Part model, mm, in its own coordinate system. Face numbers are marked on the shaded views. A direction names the side the tool comes from. Give positions to 0.01 mm unless a question says otherwise; leave off trailing zeros. Write each loop counter-clockwise with the first axis right and the second up, starting at its lowest first coordinate (ties: lowest second). Pieces come first, ordered by that corner, then holes.
```python
from build123d import *

# Parameters (mm, degrees)
PAD002_DEPTH    = 7
PAD003_DEPTH    = 3
CHAMFER003_SIZE = 1.5
SKETCH009_W     = 7.9
SKETCH009_H     = 8.3
PAD004_DEPTH    = 7.9
FILLET001_R     = 3.94
SKETCH010_R     = 1
HOLE002_DEPTH   = 25
SKETCH012_W     = 2.9
SKETCH012_H     = 8.3
PAD005_DEPTH    = 10
PAD006_DEPTH    = 8.3
FILLET002_R     = 0.5


with BuildPart() as part:
    # Sketch006 → Pad002 (new body)
    with BuildSketch(Plane.XY.offset(4)):
        Polygon((-62, 2.5), (-62, -16), (62, -16), (62, 2.5), (42, 2.5), (31.5, -8), (-31.5, -8), (-42, 2.5), align=None)
    extrude(amount=PAD002_DEPTH)

    # Sketch007 (on Face9 of Pad002) → Pad003 (join)
    with BuildSketch(Plane(origin=(0, 0, 4), x_dir=(1, 0, 0), z_dir=(0, 0, -1))):
        with BuildLine():
            Line((-31.5, 8), (31.5, 8))
            Line((37.293259, 2.206741), (31.5, 8))
            Line((38.566051, 3.479533), (37.293259, 2.206741))
            Line((32.772792, 9.272792), (38.566051, 3.479533))
            ThreePointArc((32.772792, 9.272792), (32.18883, 9.662983), (31.5, 9.8))
            Line((31.5, 9.8), (-31.5, 9.8))
            ThreePointArc((-31.5, 9.8), (-32.18883, 9.662983), (-32.772792, 9.272792))
            Line((-38.566051, 3.479533), (-32.772792, 9.272792))
            Line((-37.293259, 2.206741), (-38.566051, 3.479533))
            Line((-31.5, 8), (-37.293259, 2.206741))
        make_face()
    extrude(amount=PAD003_DEPTH)

    # Chamfer003
    chamfer003_edges = [part.edges().sort_by_distance(p)[0] for p in [
        (-35.669422, -6.376163, 4),
    ]]
    chamfer(chamfer003_edges, length=CHAMFER003_SIZE)

    # Sketch009 (on Face1 of Chamfer003) → Pad004 (join)
    with BuildSketch(Plane(origin=(0, 0, 4), x_dir=(1, 0, 0), z_dir=(0, 0, -1))):
        with Locations((-58.05, 6.75)):
            Rectangle(SKETCH009_W, SKETCH009_H)
    extrude(amount=PAD004_DEPTH)

    # Fillet001
    fillet001_edges = [part.edges().sort_by_distance(p)[0] for p in [
        (-54.1, -6.75, -3.9),
        (-62, -6.75, -3.9),
    ]]
    fillet(fillet001_edges, radius=FILLET001_R)

    # Sketch010 (on Face1 of Fillet001) → Hole002 (cut)
    with BuildSketch(Plane.XZ.offset(10.9)):
        with Locations((-58, 0)):
            Circle(SKETCH010_R)
    extrude(amount=-HOLE002_DEPTH, mode=Mode.SUBTRACT)

    # Sketch012 (on Face4 of Hole002) → Pad005 (join)
    with BuildSketch(Plane(origin=(0, 0, 4), x_dir=(1, 0, 0), z_dir=(0, 0, -1))):
        with Locations((60.55, 6.75)):
            Rectangle(SKETCH012_W, SKETCH012_H)
    extrude(amount=PAD005_DEPTH)

    # Sketch013 (on Face21 of Pad005) → Pad006 (join)
    with BuildSketch(Plane.XZ.offset(10.9)):
        Polygon((59.1, -6), (57.2, -2.1), (59.1, -2.1), align=None)
    extrude(amount=-PAD006_DEPTH)

    # Fillet002
    fillet002_edges = [part.edges().sort_by_distance(p)[0] for p in [
        (57.2, -6.75, -2.1),
    ]]
    fillet(fillet002_edges, radius=FILLET002_R)


solid = part.part
```
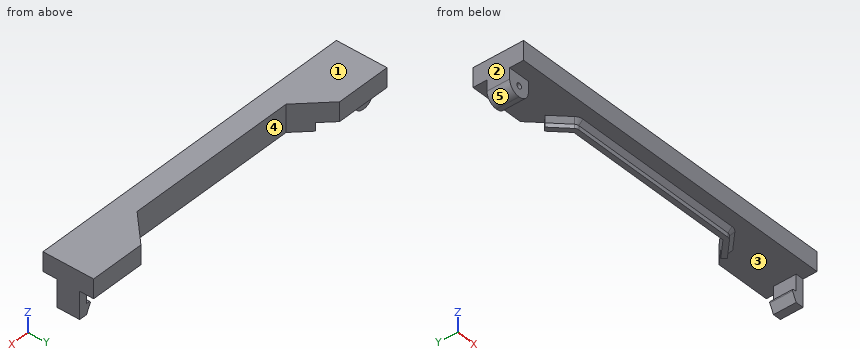
1) Pin check, flat tips, straight feed: pin 1 Ø3 at (y, z) = (-3, -3.5) entering from -X; pin 2 Ø4 at (x, z) = (-59.5, 1.5) entering from +Y; pin 3 Ø6 at (x, z) = (-35.5, 1) entering from +Y. Stop position of each tip, or through.
Answers follow:
pin 1: stops at x = -61.43
pin 2: stops at y = -2.6
pin 3: stops at y = -2.21
2) Wall check: L1, parallel to Z at x = -58, y = -4.25; L2, parallel to Y at x = -23.5, z = 9; L3, parallel to X at y = -7, z = 4.25. Give the ranges that are in metal, low to high.
Answers follow:
L1: z = -3.9 to -1, 1 to 11
L2: y = -16 to -8
L3: x = -62 to -32.5, 32.5 to 62
3) Saw through at D-D, the plane x = -47.5. Write the cut outline in (y, z), then the cut area to 4 significant figures.
Answers follow:
outline: (-16, 4) - (2.5, 4) - (2.5, 11) - (-16, 11) - close
area: 129.5 mm2
4) 3-axis set-ups, long thin cutter, end or side, ignore diameter. For the marked faces 4 and 5: which of +Z, -Z, +X, -X, +Y, -Y reach the whole face in a straight line?
Answers follow:
face 4: +Z, -Z, +Y
face 5: -Z, -X, +Y, -Y
5) Two-plate mould, pull along X, no slides. Class the marked faces 1, 2 and 3: +X half, -X half, draft (parallel to the pull), parting line (faces both ways), or undercut.
Answers follow:
face 1: draft
face 2: -X half
face 3: undercut
6) Saw through at A-A, the plane y = 1. Write the cut outline in (x, z).
Answers follow:
outline: (-62, 4) - (-40.5, 4) - (-40.5, 11) - (-62, 11) - close; (40.5, 4) - (62, 4) - (62, 11) - (40.5, 11) - close
7) Saw through at C-C, the plane y = -14. Write the cut outline in (x, z).
Answers follow:
outline: (-62, 4) - (62, 4) - (62, 11) - (-62, 11) - close
8) Saw through at B-B, the plane x = 22.5. Write the cut outline in (y, z), then the cut area to 3 significant figures.
Answers follow:
outline: (-16, 4) - (-11.3, 4) - (-9.8, 2.5) - (-9.8, 1) - (-8, 1) - (-8, 11) - (-16, 11) - close
area: 62.5 mm2
